Autodesk Fusion 360 part; units mm, degrees
sketch "Sketch1" plane through (0, 0, 0) normal (0, 0, 1) x (1, 0, 0)
  line L0 (0, 0) -> (13, 0)
  line L1 (13, 0) -> (13, 40)
  line L2 (13, 40) -> (0, 40)
  line L3 (0, 40) -> (0, 0)
  dimension "d1" = 13
  dimension "d2" = 40
extrude "Extrude1" add sketch "Sketch1" along normal blind 7 and the other way blind 0
sketch "Sketch2" plane through (0, 0, 0) normal (0, -1, 0) x (1, 0, 0)
  line L0 (0, 0) -> (13, 0)
  line L1 (13, 0) -> (13, 7)
  line L2 (13, 7) -> (0, 7)
  line L3 (0, 7) -> (0, 0)
  circle A0 centre (8.6106, 7) radius 4.1
  dimension "d5" = 8.2
extrude "Extrude2" cut sketch "Sketch2" against normal blind 41 contours L2 A0 picked at (8.104, 4.6437)
sketch "Sketch4" plane through (0, 0, 7) normal (0, 0, 1) x (-1, 0, 0)
  line L0 (-4.5106, 0) -> (-4.5106, -40)
  line L1 (-4.5106, -40) -> (0, -40)
  line L2 (0, -40) -> (0, 0)
  line L3 (0, 0) -> (-4.5106, 0)
  line L4 (-0.517, -40) -> (-1.5, -40)
  line L5 (-1.5, -40) -> (-1.5, 0)
  line L6 (-1.5, 0) -> (-0.517, 0)
  line L7 (-0.517, 0) -> (-0.517, -40)
extrude "Extrude4" cut sketch "Sketch4" against normal blind 6.5 contours L1 L3 L4 L5 L6 L7
sketch "Sketch5" plane through (0, 0, 0) normal (-1, 0, 0) x (0, -1, 0)
  line L0 (-40, 0) -> (0, 0)
  line L1 (0, 0) -> (0, 7)
  line L2 (0, 7) -> (-40, 7)
  line L3 (-40, 7) -> (-40, 0)
  circle A0 centre (-20, 3.9772) radius 3.5
  line L4 (-23.5, 3.9917) -> (-23.4875, 7)
  line L5 (-16.5, 3.9917) -> (-16.5125, 7)
  dimension "d15" = 7
extrude "Extrude5" cut sketch "Sketch5" against normal blind 1 contours L2 A0 L4 | L2 A0 L5 | L2 A0 picked at (-19.7165, 7.2777)
Could you check a few things on this model? Use its own coordinates, in mm. A direction names the side the tool comes from. Coordinates: 2 decimals unless noted, no trailing zeros. Loops run counter-clockwise (first coordinate to the right, second up) from the corner with the lowest first, then second, coordinate; pieces in that order, holes last.
1. I need wall thicknesses on L1, parallel to X at y = 27, z = 6.75; L2, parallel to X at y = 28, z = 2; L3, parallel to X at y = 9.5, z = 3.5. Which ranges of each line are inside material? Lowest first, please.
2. We'd pull the mould along X, two halves only. Please class faces 3 (the face through (1, 20, 0.5)), 4 (the face through (8.5, 19.7, 2.9)), 5 (the face through (0, 20, 3)), 6 (the face through (3, 20, 7)): released by +X, released by -X, zero draft, split by the parting line, or undercut.
3. Imagine slicing it at A-A (z = 1.75). Please give me the cut outline in (x, y).
4. Imagine slicing it at C-C (z = 5.5). Please give me the cut outline in (x, y), and give its area (3 significant figures).
5. For P1, Ø0.8, axis at x = 1, y = 10.5, coming from the +Z side, with a flat end and sliding along its axis, tell me the tip position at first contact or that it passes through.
6. For faces 1 (the face through (13, 20, 3)), 2 (the face through (1.5, 20, 4)), which set-ups out of +Z, -Z, +X, -X, +Y, -Y let a thin tool reach every point of the face, with its end or its side?
7. Imagine slicing it at B-B (y = 35). Please give me the cut outline in (x, z).
8. Imagine slicing it at D-D (z = 3.25). Please give me the cut outline in (x, y).
Computed values:
1. L1: x = 0 to 0.52, 1.5 to 4.52, 12.7 to 13
1. L2: x = 0 to 0.52, 1.5 to 13
1. L3: x = 0 to 0.52, 1.5 to 6.48, 10.75 to 13
2. face 3: undercut
2. face 4: undercut
2. face 5: released by -X
2. face 6: zero draft
3. outline: (0, 0) - (0.52, 0) - (0.52, 40) - (0, 40) - close; (1.5, 0) - (13, 0) - (13, 40) - (1.5, 40) - close
4. outline: (0, 0) - (0.52, 0) - (0.52, 16.51) - (0, 16.51) - close; (0, 16.85) - (0.52, 16.85) - (0.52, 23.15) - (0, 23.15) - close; (0, 23.49) - (0.52, 23.49) - (0.52, 40) - (0, 40) - close; (1.5, 0) - (4.79, 0) - (4.79, 40) - (1.5, 40) - close; (12.43, 0) - (13, 0) - (13, 40) - (12.43, 40) - close
4. area: 175 mm2
5. P1: stops at z = 0.5
6. face 1: +Z, -Z, +X, +Y, -Y
6. face 2: +Z, +Y, -Y
7. outline: (0, 0) - (13, 0) - (13, 7) - (12.71, 7) arc R4.1 cw to (4.51, 7) - (1.5, 7) - (1.5, 0.5) - (0.52, 0.5) - (0.52, 7) - (0, 7) - close
8. outline: (0, 0) - (0.52, 0) - (0.52, 40) - (0, 40) - close; (1.5, 0) - (6.95, 0) - (6.95, 40) - (1.5, 40) - close; (10.27, 0) - (13, 0) - (13, 40) - (10.27, 40) - close
